from build123d import *

# Parameters (mm, degrees)
F0_R     = 8.25
F0_R_2   = 6.75
F1_DEPTH = 31.75
F2_R     = 8.076927
F3_DEPTH = 2
F4_R     = 5
F5_DEPTH = 25


with BuildPart() as f1:
    # F0 (on Top) → F1 (new body)
    with BuildSketch(Plane.XY):
        Circle(F0_R)
        Circle(F0_R_2, mode=Mode.SUBTRACT)
    extrude(amount=F1_DEPTH)

    # F2 (on Top) → F3 (join)
    with BuildSketch(Plane.XY):
        Circle(F2_R)
    extrude(amount=F3_DEPTH)

    # F4 (on face) → F5 (cut)
    with BuildSketch(Plane(origin=(0, 0, 0), x_dir=(1, 0, 0), z_dir=(0, 0, -1))):
        Circle(F4_R)
    extrude(amount=-F5_DEPTH, mode=Mode.SUBTRACT)


solid = f1.part
The model under review builds one solid part; all positions refer to its coordinate system, in mm. A direction names the side the tool comes from. Round coordinates to 2 decimals unless told otherwise and drop trailing zeros. Write each loop counter-clockwise with the first axis right and the second up, starting at its lowest first coordinate (ties: lowest second). Pieces come first, ordered by that corner, then holes. Notation, with made-up numbers: M 65,51 L 90,51 A15 cw 90,75 Z; hole C 84,-21 d3. An arc over 180 degrees is marked long. Use a Markdown table: item, result. Add a question column.
Q1. Machinability: for faces 4 (the face through (-1.08, 4.88, 0.99)), 5 (the face through (-5, -2, 2)), which of the approach directions +Z, -Z, +X, -X, +Y, -Y give a long, thin tool a straight path to every point of the face, cutting with its end or side? Answer none if there is none.
Q2. We need section A-A, the plane y = 0. State the section outline as (x, z) points, plus the area to 3 significant figures.
Q3. We need section D-D, the plane y = -6. State the section outline as (x, z) points, plus the area to 3 significant figures.
Q4. We need section C-C, the plane z = 19. State the section outline as (x, y) points.
Q5. The part is to be moulded in two halves that separate along Y. For faces 1 (the face through (-7, 0, 31.75)), 2 (the face through (-1.46, -6.59, 16.67)), 3 (the face through (7.62, -3.16, 15.65)), say which applies: pulls with the +Y half, pulls with the -Y half, needs draft (parallel to the pull), parting line crosses it, or undercut.
Q6. To check wall thickness, follow line 1 (Y direction, x = 0, z = 0.65); line 2 (Z direction, x = -4.5, y = -5); line 3 (Y direction, x = 5.25, z = 18.5). State the ranges of each line that lie inside material, in increasing order.
Q7. Insertion check: pin 1 (2 mm diameter, centred on x = -3, z = 19.5, fed in from +Y); pin 2 (1.5 mm diameter, centred on y = -4, z = 24.5, fed in from +X); pin 3 (1 mm diameter, centred on x = 3, z = 23, fed in from -Y). Each pin has a flat end and moves straight along its axis. Give the tip position at first contact, or say it passes through.
Findings below:
| question | item | result |
|---|---|---|
| 1 | face 4 | +Z, -Z |
| 1 | face 5 | +Z |
| 2 | outline | M -8.25,0 L -5,0 L -5,2 L -6.75,2 L -6.75,31.75 L -8.25,31.75 Z; M 5,0 L 8.25,0 L 8.25,31.75 L 6.75,31.75 L 6.75,2 L 5,2 Z |
| 2 | area | 102 mm² |
| 3 | outline | M -5.66,0 L 5.66,0 L 5.66,31.75 L 3.09,31.75 L 3.09,2 L -3.09,2 L -3.09,31.75 L -5.66,31.75 Z |
| 3 | area | 176 mm² |
| 4 | outline | C 0,0 d16.5; hole C 0,0 d13.5 |
| 5 | face 1 | needs draft |
| 5 | face 2 | undercut |
| 5 | face 3 | parting line crosses it |
| 6 | line 1 | y = -8.25 to -5, 5 to 8.25 |
| 6 | line 2 | z = 0 to 2 |
| 6 | line 3 | y = -6.36 to -4.24, 4.24 to 6.36 |
| 7 | pin 1 | stops at y = 8 |
| 7 | pin 2 | stops at x = 7.58 |
| 7 | pin 3 | stops at y = -7.86 |
